Autodesk Inventor part; units mm, degrees
ref_plane "YZ Plane" through (0, 0, 0) normal (1, 0, 0) x (0, 1, 0)
ref_plane "XZ Plane" through (0, 0, 0) normal (0, 1, 0) x (-1, 0, 0)
ref_plane "XY Plane" through (0, 0, 0) normal (0, 0, 1) x (1, 0, 0)
sketch "Sketch3" plane through (0, 0, 0) normal (0, 0, 1) x (1, 0, 0)
  line L0 (0, 0) -> (812.8, 0) construction
  line L1 (812.8, 0) -> (812.8, -406.4) construction
  line L2 (812.8, -406.4) -> (0, -406.4) construction
  line L3 (0, -406.4) -> (0, 0) construction
  line L4 (406.4, 0) -> (0, 0)
  line L5 (0, -406.4) -> (0, 0)
  line L6 (0, -406.4) -> (406.4, -406.4)
  line L7 (406.4, 0) -> (406.4, -406.4)
  dimension "d88" = 812.8
extrude "Extrusion2" add sketch "Sketch3" against normal blind 406.4
sketch "Sketch4" plane through (0, 0, 0) normal (0, 0, 1) x (1, 0, 0)
  line L0 (0, 0) -> (406.4, 0)
  line L1 (0, 0) -> (812.8, 0) construction
  line L2 (812.8, 0) -> (812.8, -406.4) construction
  line L3 (812.8, -406.4) -> (0, -406.4) construction
  line L4 (0, -406.4) -> (0, 0) construction
  line L5 (0, 0) -> (25.4, 0)
  line L6 (25.4, 0) -> (25.4, -25.4)
  line L7 (25.4, -25.4) -> (0, -25.4)
  line L8 (0, -25.4) -> (0, 0)
  line L9 (25.4, -25.4) -> (381, -25.4)
  line L10 (381, -25.4) -> (381, -381)
  line L11 (381, -381) -> (25.4, -381)
  line L12 (25.4, -381) -> (25.4, -25.4)
  dimension "d95" = 812.8
  dimension "d102" = 25.4
  dimension "d103" = 25.4
  dimension "d104" = 355.6
  dimension "d105" = 355.6
extrude "Extrusion3" cut sketch "Sketch4" against normal blind 406.4 contours L9 L10 L11 L12
sketch "Sketch5" plane through (0, -406.4, 0) normal (-1, 0, 0) x (0, 0, 1)
  line L0 (0, 406.4) -> (-406.4, 406.4)
  line L1 (-406.4, 406.4) -> (-381, 406.4)
  line L2 (-381, 406.4) -> (-381, 381)
  line L3 (-381, 381) -> (-406.4, 381)
  line L4 (-406.4, 381) -> (-406.4, 406.4)
  line L5 (-381, 381) -> (-25.4, 381)
  line L6 (-25.4, 381) -> (-25.4, 25.4)
  line L7 (-25.4, 25.4) -> (-381, 25.4)
  line L8 (-381, 25.4) -> (-381, 381)
  dimension "d108" = 25.4
  dimension "d109" = 25.4
  dimension "d110" = 355.6
  dimension "d111" = 355.6
extrude "Extrusion4" cut sketch "Sketch5" against normal blind 406.4 contours L5 L6 L7 L8
sketch "Sketch6" plane through (0, 0, 0) normal (0, 1, 0) x (1, 0, 0)
  line L0 (0, 406.4) -> (406.4, 406.4)
  line L1 (0, 406.4) -> (25.4, 406.4)
  line L2 (25.4, 406.4) -> (25.4, 381)
  line L3 (25.4, 381) -> (0, 381)
  line L4 (0, 381) -> (0, 406.4)
  line L5 (25.4, 381) -> (381, 381)
  line L6 (381, 381) -> (381, 25.4)
  line L7 (381, 25.4) -> (25.4, 25.4)
  line L8 (25.4, 25.4) -> (25.4, 381)
  point P0 (0, 0)
  dimension "d114" = 25.4
  dimension "d115" = 25.4
  dimension "d116" = 355.6
  dimension "d117" = 355.6
extrude "Extrusion5" cut sketch "Sketch6" against normal blind 406.4 contours L5 L6 L7 L8
properties part number "JukeBox Metal Frame"
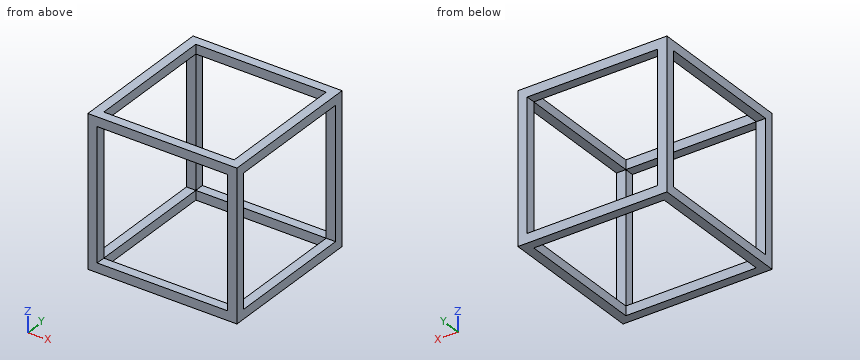
The listing builds one solid part. Answer for the finished solid, in the listing's coordinates (mm). Round coordinates to 2 decimals unless told otherwise and drop trailing zeros. Write each loop counter-clockwise with the first axis right and the second up, starting at its lowest first coordinate (ties: lowest second). Pieces come first, ordered by that corner, then holes. Notation, with made-up numbers: (50.5, -19) - (104.5, -19) arc R12 ccw to (104.5, 2) - close; hole circle Ø2 at (47.5, -32.5). An arc over 180 degrees is marked (long way). Use a Markdown table: item, result. Add a question column.
1. The part is cut by section B-B (x = 116). Write down the section's boundary in (y, z), and give its area (3 significant figures).
2. Consider line 1 (X direction, y = -111, z = -16.5); line 2 (Y direction, x = 384, z = -89.5). Determine where each line is inside the solid, lowest interval first.
3. The part is cut by section A-A (y = -41.5). Write down the section's boundary in (x, z), and give its area (3 significant figures).
Reported:
| question | item | result |
|---|---|---|
| 1 | outline | (-406.4, -406.4) - (-381, -406.4) - (-381, -381) - (-406.4, -381) - close; (-406.4, -25.4) - (-381, -25.4) - (-381, 0) - (-406.4, 0) - close; (-25.4, -406.4) - (0, -406.4) - (0, -381) - (-25.4, -381) - close; (-25.4, -25.4) - (0, -25.4) - (0, 0) - (-25.4, 0) - close |
| 1 | area | 2,580 mm^2 |
| 2 | line 1 | 0 to 25.4, 381 to 406.4 |
| 2 | line 2 | -406.4 to -381, -25.4 to 0 |
| 3 | outline | (0, -406.4) - (25.4, -406.4) - (25.4, -381) - (0, -381) - close; (0, -25.4) - (25.4, -25.4) - (25.4, 0) - (0, 0) - close; (381, -406.4) - (406.4, -406.4) - (406.4, -381) - (381, -381) - close; (381, -25.4) - (406.4, -25.4) - (406.4, 0) - (381, 0) - close |
| 3 | area | 2,580 mm^2 |
